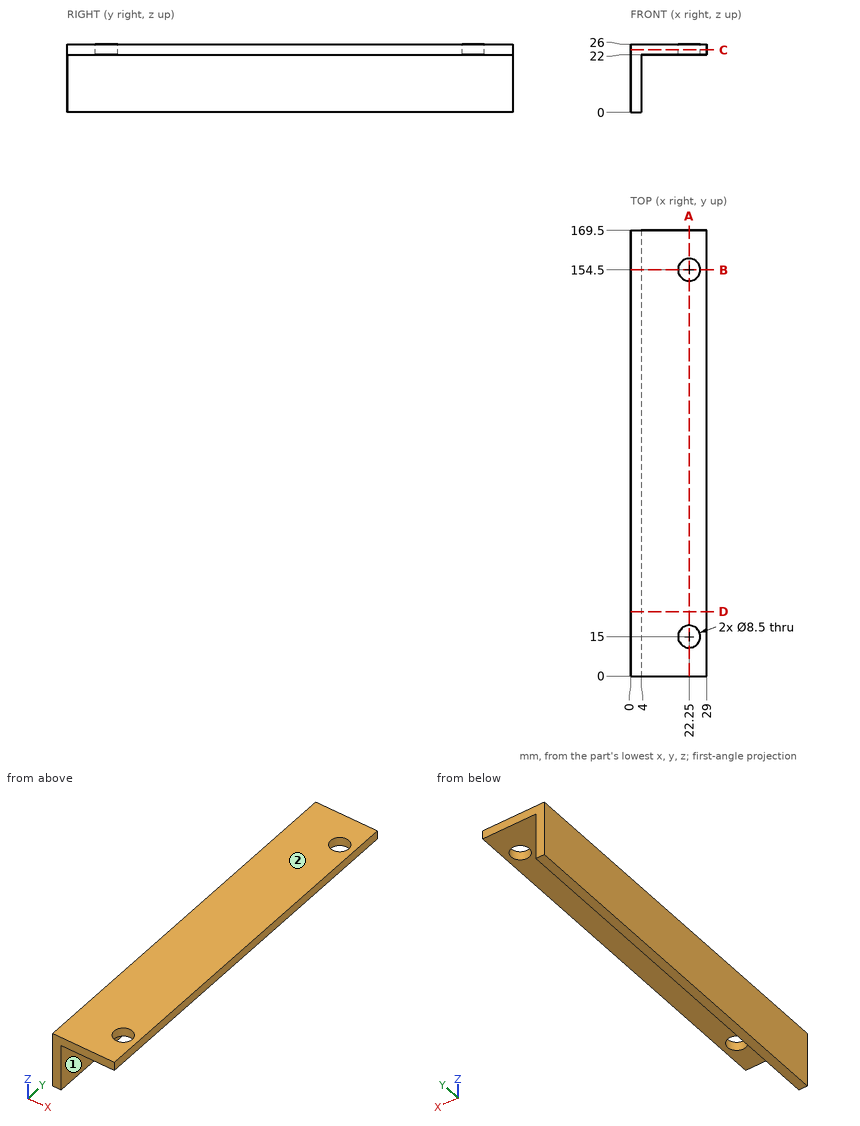
The drawing under review shows one solid part. Ordinate dimensions are in mm from its lowest x, y, z. A direction names the side the tool comes from. Round coordinates to 2 decimals unless told otherwise and drop trailing zeros. Loops run counter-clockwise (first coordinate to the right, second up) from the corner with the lowest first, then second, coordinate; pieces in that order, holes last. Notation, with made-up numbers: (56, -18) -> (84, -18) arc R28 cw to (84, 14) -> close; hole circle Ø10 at (65, -33). An arc over 180 degrees is marked (long way). One line per question, with ' | ' between items. Start each with the question number.
Item 1: Machinability: for the marked faces 1 and 2, which of the approach directions +Z, -Z, +X, -X, +Y, -Y give a long, thin tool a straight path to every point of the face, cutting with its end or side? Answer none if there is none.
Item 2: Wall thickness on line 1 along Y through (x, z) = (22.25, 23.85); line 2 along Z through (x, y) = (25.5, 150.5); line 3 along X through (y, z) = (154, 23.5): over which ranges is each line inside the solid? List them lowest first. Write a range as [from, to].
Item 3: Add section C-C, the plane z = 23.75. Write out the cut boundary in (x, y).
Item 4: Add section D-D, the plane y = 24.5. Write out the cut boundary in (x, z).
Item 5: Add section A-A, the plane x = 22.25. Write out the cut boundary in (y, z).
Item 6: Add section B-B, the plane y = 154.5. Write out the cut boundary in (x, z), then the cut area to 3 significant figures.
Item 7: For pin 1 (10 mm diameter, centred on y = 106.5, z = 15.5, fed in from +X); pin 2 (13.5 mm diameter, centred on x = 22.25, y = 15, fed in from -Z); pin 3 (7 mm diameter, centred on x = 22.25, y = 154.5, fed in from -Z), all flat-tipped, find the tip position at first contact; note any pin that passes through.
Return value:
1) face 1: -Z, +X, +Y, -Y | face 2: +Z, +X, -X, +Y, -Y
2) line 1: y = [0, 10.75], [19.25, 150.25], [158.75, 169.5] | line 2: z = [22, 26] | line 3: x = [0, 18.03], [26.47, 29]
3) outline: (0, 0) -> (29, 0) -> (29, 169.5) -> (0, 169.5) -> close; hole circle Ø8.5 at (22.25, 15); hole circle Ø8.5 at (22.25, 154.5)
4) outline: (0, 0) -> (4, 0) -> (4, 22) -> (29, 22) -> (29, 26) -> (0, 26) -> close
5) outline: (0, 22) -> (10.75, 22) -> (10.75, 26) -> (0, 26) -> close; (19.25, 22) -> (150.25, 22) -> (150.25, 26) -> (19.25, 26) -> close; (158.75, 22) -> (169.5, 22) -> (169.5, 26) -> (158.75, 26) -> close
6) outline: (0, 0) -> (4, 0) -> (4, 22) -> (18, 22) -> (18, 26) -> (0, 26) -> close; (26.5, 22) -> (29, 22) -> (29, 26) -> (26.5, 26) -> close | area: 170 mm2
7) pin 1: stops at x = 4 | pin 2: stops at z = 22 | pin 3: passes through
